from build123d import *

# Parameters (mm, degrees)
F0_W     = 304.8
F0_H     = 50.8
F0_R     = 6.35
F1_DEPTH = 19.05


# Not quite as in the source:
# - a pattern or mirror of a feature is missing from the dataset's text; its kind, count and spacing are read off the source's solid


with BuildPart() as f1:
    # F0 (on Front) → F1 (new body)
    with BuildSketch(Plane.XZ):
        Rectangle(F0_W, F0_H)
        Circle(F0_R, mode=Mode.SUBTRACT)
    extrude(amount=F1_DEPTH)

    # F1_copies: F1 across plane


with BuildPart() as f1_1:
    add(f1.part)
    add(f1.part.mirror(Plane(origin=(0, -12.7, 0), x_dir=(0, 0, -1), z_dir=(0, -1, 0))))


solid = f1_1.part
Build history of the part. All positions in model axes, mm. Give positions to 0.01 mm unless a question says otherwise; leave off trailing zeros. Order: outer loops, then holes, each group sorted by start corner. A loop starts at its lowest first (then second) coordinate and runs counter-clockwise, first axis right, second up. Notation, with made-up numbers: M 27,11.25 L 82,11.25 A15 ccw 82,20.25 Z; hole C 35,70.5 d8. An arc over 180 degrees is marked long. Use one line per item in the form item = value.
Q1. Slice it at B-B, the plane z = 0. Write the cut outline in (x, y), and give its area (3 significant figures).
Conclusion:
outline = M -152.4,-25.4 L -6.35,-25.4 L -6.35,0 L -152.4,0 Z; M 6.35,-25.4 L 152.4,-25.4 L 152.4,0 L 6.35,0 Z
area = 7,420 mm2
Q2. Pin check, flat tip, straight feed: P1, Ø10, axis at x = 0, z = 0, coming from the +Y side. Stop position of the tip, or through.
Conclusion:
P1 = through
Q3. Wall check: probe 1 along Z at (x, y) = (0, -18.5); probe 2 along X at (y, z) = (-16.5, 5.5). Give the ranges that are in metal, low to high.
Conclusion:
probe_1 = -25.4 to -6.35, 6.35 to 25.4
probe_2 = -152.4 to -3.17, 3.17 to 152.4
Q4. Slice it at A-A, the plane x = 0. Write the cut outline in (y, z), and give its area (3 significant figures).
Conclusion:
outline = M -25.4,-25.4 L 0,-25.4 L 0,-6.35 L -25.4,-6.35 Z; M -25.4,6.35 L 0,6.35 L 0,25.4 L -25.4,25.4 Z
area = 968 mm2
Q5. Pull direction Z, two halves, no side cores. Call faces 1 (the flat face through (152.4, -13, 0)), 2 (the flat face through (-2, -13, -25.4)), 3 (the cylindrical face through (-1.38, -12.52, -6.2)): released by +Z, released by -Z, zero draft, split by the parting line, or undercut.
Conclusion:
face_1 = zero draft
face_2 = released by -Z
face_3 = undercut
